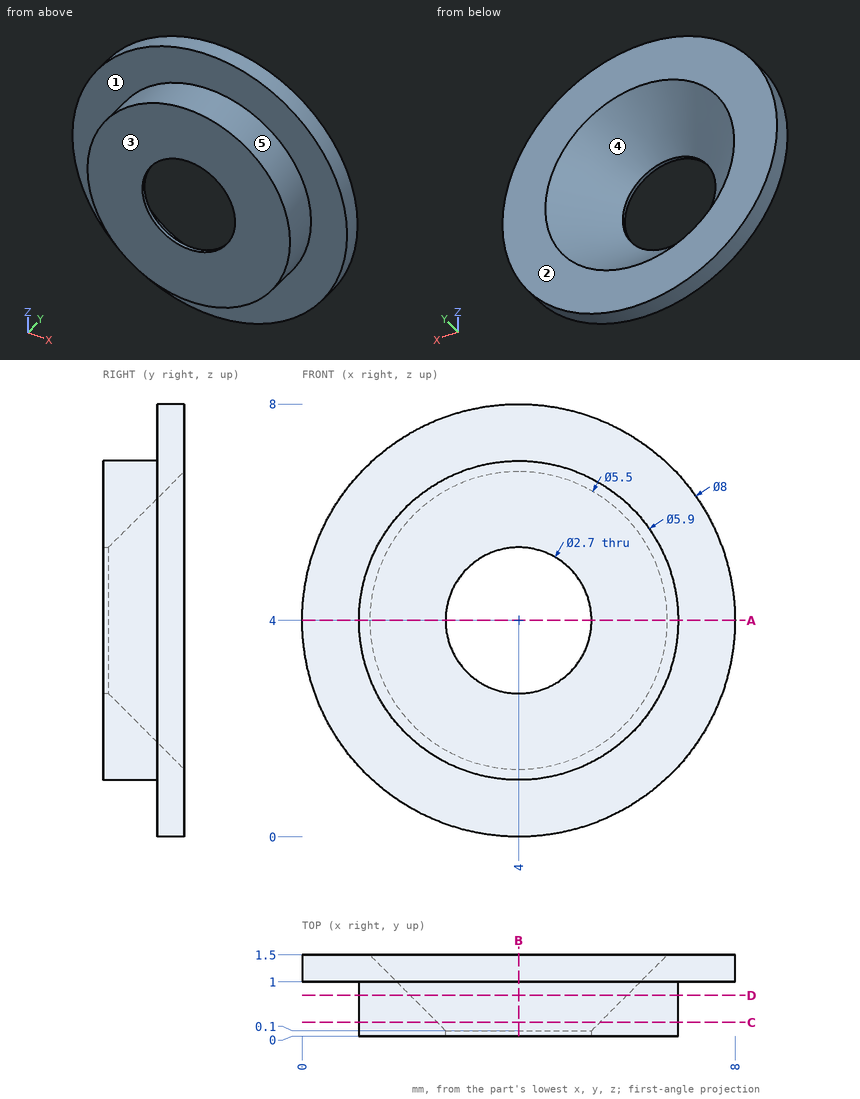
For this review, use the dimensioned drawing (mm, ordinates from the lowest corner) and the shaded views. A direction names the side the tool comes from. Round coordinates to 2 decimals unless told otherwise and drop trailing zeros. Order: outer loops, then holes, each group sorted by start corner. A loop starts at its lowest first (then second) coordinate and runs counter-clockwise, first axis right, second up. Notation, with made-up numbers: (58, -5) -> (97, -5) arc R11 ccw to (97, 14) -> close; hole circle Ø10 at (61.5, 42.5). An arc over 180 degrees is marked (long way). Put each result on its own line as item: value.
Q1. Add section D-D on y = 0.75. Write out the cut boundary in (x, z).
Check result:
outline: circle Ø5.9 at (4, 4); hole circle Ø4 at (4, 4)
Q2. Add section C-C on y = 0.25. Write out the cut boundary in (x, z), plus the area to 3 significant figures.
Check result:
outline: circle Ø5.9 at (4, 4); hole circle Ø3 at (4, 4)
area: 20.3 mm2
Q3. Insertion check: pin 1 Ø2.5 at (x, z) = (4, 4) entering from +Y. The pin has a flat end and moves straight along its axis. Give the tip position at first contact, or say it passes through.
Check result:
pin 1: through
Q4. Add section B-B on x = 4. Write out the cut boundary in (y, z).
Check result:
outline: (0, 1.05) -> (1, 1.05) -> (1, 0) -> (1.5, 0) -> (1.5, 1.25) -> (0.1, 2.65) -> (0, 2.65) -> close; (0, 5.35) -> (0.1, 5.35) -> (1.5, 6.75) -> (1.5, 8) -> (1, 8) -> (1, 6.95) -> (0, 6.95) -> close
Q5. Add section A-A on z = 4. Write out the cut boundary in (x, y), plus the area to 3 significant figures.
Check result:
outline: (0, 1) -> (1.05, 1) -> (1.05, 0) -> (2.65, 0) -> (2.65, 0.1) -> (1.25, 1.5) -> (0, 1.5) -> close; (5.35, 0) -> (6.95, 0) -> (6.95, 1) -> (8, 1) -> (8, 1.5) -> (6.75, 1.5) -> (5.35, 0.1) -> close
area: 3.89 mm2
Q6. For probe 1 along X at (y, z) = (0.05, 4); probe 2 along X at (y, z) = (0.8, 5.5); probe 3 along Z at (x, y) = (4.25, 0.6), list the stretches that pass through material, from the lowest coordinate up. Write a range as [from, to].
Check result:
probe 1: [1.05, 2.65], [5.35, 6.95]
probe 2: [1.46, 2.6], [5.4, 6.54]
probe 3: [1.06, 2.17], [5.83, 6.94]
Q7. Machinability: for the marked faces 1 and 2, which of the approach directions +Z, -Z, +X, -X, +Y, -Y give a long, thin tool a straight path to every point of the face, cutting with its end or side? Answer none if there is none.
Check result:
face 1: -Y
face 2: +Z, -Z, +X, -X, +Y
Q8. Mouldability with a two-part tool opening along X and no side actions: class the marked faces 3, 4 and 5 as pulls with the +X half, pulls with the -X half, needs draft (parallel to the pull), parting line crosses it, or undercut.
Check result:
face 3: needs draft
face 4: undercut
face 5: parting line crosses it
